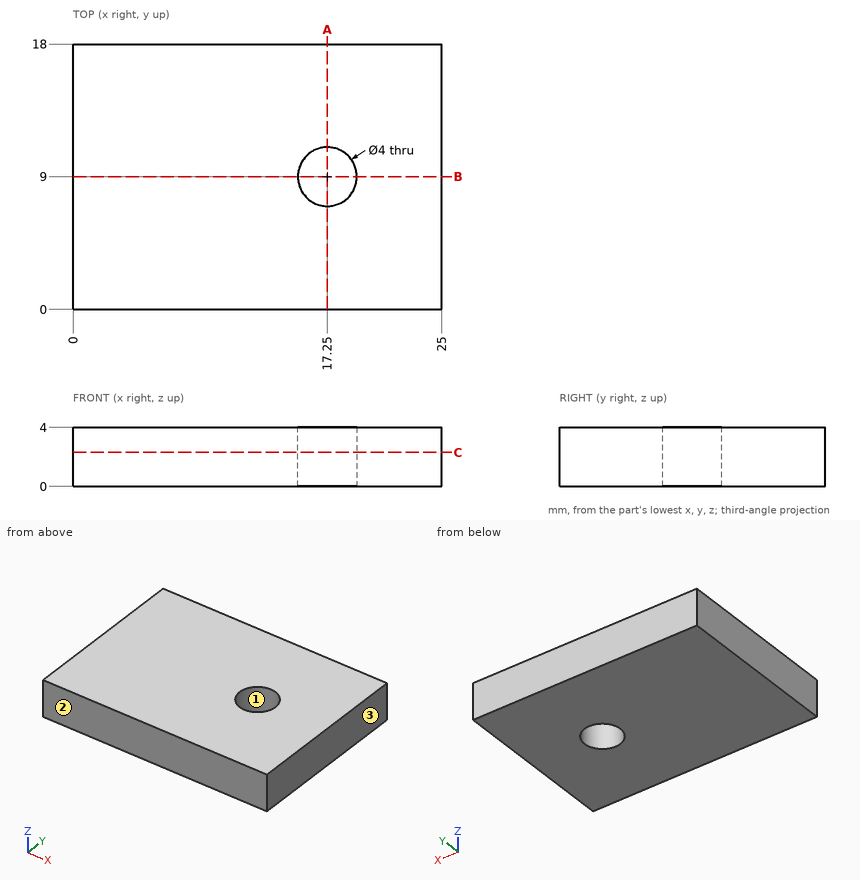
Can you work these out from the drawing? Everything is in mm from the part's minimum corner. Coordinates: 2 decimals unless noted, no trailing zeros. Loops run counter-clockwise (first coordinate to the right, second up) from the corner with the lowest first, then second, coordinate; pieces in that order, holes last. Notation, with made-up numbers: M 23,17.25 L 32,17.25 A25 ccw 32,49.25 Z; hole C 18,-24.5 d3. An arc over 180 degrees is marked long. One line per item, written item: value.
1. Imagine slicing it at C-C (z = 2.3). List the corners of the cut face in (x, y) for me, and give its area (3 significant figures).
Geometry says:
outline: M 0,0 L 25,0 L 25,18 L 0,18 Z; hole C 17.25,9 d4
area: 437 mm2
2. Thinking about a two-plate mould opening in Y: for the marked faces 1, 2 and 3, which applies, +Y half, -Y half, draft (parallel to the pull), parting line (faces both ways), or undercut?
Geometry says:
face 1: undercut
face 2: -Y half
face 3: draft
3. Please list where these lines run through material, in increasing order: probe 1 along Y at (x, z) = (17.25, 1.35); probe 2 along X at (y, z) = (7.5, 3.4); probe 3 along Y at (x, z) = (16, 3.1).
Geometry says:
probe 1: y = 0 to 7, 11 to 18
probe 2: x = 0 to 15.93, 18.57 to 25
probe 3: y = 0 to 7.44, 10.56 to 18
4. Imagine slicing it at B-B (y = 9). List the corners of the cut face in (x, z) for me.
Geometry says:
outline: M 0,0 L 15.25,0 L 15.25,4 L 0,4 Z; M 19.25,0 L 25,0 L 25,4 L 19.25,4 Z
5. Imagine slicing it at A-A (x = 17.25). List the corners of the cut face in (y, z) for me.
Geometry says:
outline: M 0,0 L 7,0 L 7,4 L 0,4 Z; M 11,0 L 18,0 L 18,4 L 11,4 Z
